```python
from build123d import *

# Parameters (mm, degrees)
SZKIC1_R                    = 1.5
SZKIC1_R_2                  = 1.6
DODANIE_WYCI_GNI_CIE1_DEPTH = 20
ZAOKR_GLENIE1_R             = 3
SFAZOWANIE1_SIZE            = 1
SZKIC2_R                    = 1.5
SZKIC2_R_2                  = 1.6
DODANIE_WYCI_GNI_CIE2_DEPTH = 0.2


with BuildPart() as part:
    # Szkic1 → Dodanie-wyciągnięcie1 (new body)
    with BuildSketch(Plane.XY):
        Polygon((-39.009773604, 35.733555733), (-39.009773604, 39.983555733), (9.235464557, 39.983555733), (9.235464557, 35.733555733), (9.235464557, -13.466444267), (9.235464557, -17.716444267), (-39.009773604, -17.716444267), (-39.009773604, -13.466444267), align=None)
        with Locations((5.112845476, 11.133555733)):
            Circle(SZKIC1_R, mode=Mode.SUBTRACT)
        with Locations((-34.887154524, 11.133555733)):
            Circle(SZKIC1_R, mode=Mode.SUBTRACT)
        with Locations((6.285464557, -13.466444267)):
            Circle(SZKIC1_R, mode=Mode.SUBTRACT)
        with Locations((6.285464557, 35.733555733)):
            Circle(SZKIC1_R_2, mode=Mode.SUBTRACT)
        with Locations((-36.059773604, 35.733555733)):
            Circle(SZKIC1_R, mode=Mode.SUBTRACT)
        with Locations((-36.059773604, -13.466444267)):
            Circle(SZKIC1_R, mode=Mode.SUBTRACT)
        with BuildLine():
            Line((-14.087154524, -13.391444267), (-14.087154524, -12.891444267))
            Line((-14.087154524, -12.891444267), (-3.372154524, -12.891444267))
            ThreePointArc((-3.372154524, -12.891444267), (-1.675098249, -12.188500541), (-0.972154524, -10.491444267))
            Line((-0.972154524, -10.491444267), (-0.972154524, -0.591444267))
            Line((-0.972154524, -0.591444267), (-0.472154524, -0.591444267))
            Line((-0.472154524, -0.591444267), (-0.472154524, 1.008555733))
            Line((-0.472154524, 1.008555733), (-0.972154524, 1.008555733))
            Line((-0.972154524, 1.008555733), (-0.972154524, 21.258555733))
            Line((-0.972154524, 21.258555733), (-0.472154524, 21.258555733))
            Line((-0.472154524, 21.258555733), (-0.472154524, 22.858555733))
            Line((-0.472154524, 22.858555733), (-0.972154524, 22.858555733))
            Line((-0.972154524, 22.858555733), (-0.972154524, 28.930128609))
            ThreePointArc((-0.972154524, 28.930128609), (-1.154843646, 29.848568846), (-1.675098249, 30.627184884))
            Line((-1.675098249, 30.627184884), (-5.503525374, 34.455612008))
            ThreePointArc((-5.503525374, 34.455612008), (-6.282141411, 34.975866612), (-7.200581648, 35.158555733))
            Line((-7.200581648, 35.158555733), (-14.087154524, 35.158555733))
            Line((-14.087154524, 35.158555733), (-14.087154524, 35.658555733))
            Line((-14.087154524, 35.658555733), (-15.687154524, 35.658555733))
            Line((-15.687154524, 35.658555733), (-15.687154524, 35.158555733))
            Line((-15.687154524, 35.158555733), (-22.573727399, 35.158555733))
            ThreePointArc((-22.573727399, 35.158555733), (-23.492167637, 34.975866612), (-24.270783674, 34.455612008))
            Line((-24.270783674, 34.455612008), (-28.099210798, 30.627184884))
            ThreePointArc((-28.099210798, 30.627184884), (-28.619465402, 29.848568846), (-28.802154524, 28.930128609))
            Line((-28.802154524, 28.930128609), (-28.802154524, 22.858555733))
            Line((-28.802154524, 22.858555733), (-29.302154524, 22.858555733))
            Line((-29.302154524, 22.858555733), (-29.302154524, 21.258555733))
            Line((-29.302154524, 21.258555733), (-28.802154524, 21.258555733))
            Line((-28.802154524, 21.258555733), (-28.802154524, 1.008555733))
            Line((-28.802154524, 1.008555733), (-29.302154524, 1.008555733))
            Line((-29.302154524, 1.008555733), (-29.302154524, -0.591444267))
            Line((-29.302154524, -0.591444267), (-28.802154524, -0.591444267))
            Line((-28.802154524, -0.591444267), (-28.802154524, -10.491444267))
            ThreePointArc((-28.802154524, -10.491444267), (-28.099210798, -12.188500541), (-26.402154524, -12.891444267))
            Line((-26.402154524, -12.891444267), (-15.687154524, -12.891444267))
            Line((-15.687154524, -12.891444267), (-15.687154524, -13.391444267))
            Line((-15.687154524, -13.391444267), (-14.087154524, -13.391444267))
        make_face(mode=Mode.SUBTRACT)
    extrude(amount=DODANIE_WYCI_GNI_CIE1_DEPTH)

    # Zaokrąglenie1
    zaokr_glenie1_edges = [part.edges().sort_by_distance(p)[0] for p in [
        (-39.009773604, 39.983555733, 10),
        (9.235464557, 39.983555733, 10),
        (9.235464557, -17.716444267, 10),
        (-39.009773604, -17.716444267, 10),
    ]]
    fillet(zaokr_glenie1_edges, radius=ZAOKR_GLENIE1_R)

    # Sfazowanie1
    sfazowanie1_edges = [part.edges().sort_by_distance(p)[0] for p in [
        (3.612845476, 11.133555733, 20),
        (-36.387154524, 11.133555733, 20),
    ]]
    chamfer(sfazowanie1_edges, length=SFAZOWANIE1_SIZE)

    # Szkic2 → Dodanie-wyciągnięcie2 (add)
    with BuildSketch(Plane(origin=(0, 0, 0), x_dir=(-1, 0, 0), z_dir=(0, 0, -1))):
        with Locations((36.059773604, 35.733555733)):
            Circle(SZKIC2_R)
        with Locations((34.887154524, 11.133555733)):
            Circle(SZKIC2_R)
        with Locations((36.059773604, -13.466444267)):
            Circle(SZKIC2_R)
        with Locations((-6.285464557, 35.733555733)):
            Circle(SZKIC2_R_2)
        with Locations((-5.112845476, 11.133555733)):
            Circle(SZKIC2_R)
        with Locations((-6.285464557, -13.466444267)):
            Circle(SZKIC2_R)
    extrude(amount=-DODANIE_WYCI_GNI_CIE2_DEPTH)


solid = part.part
```
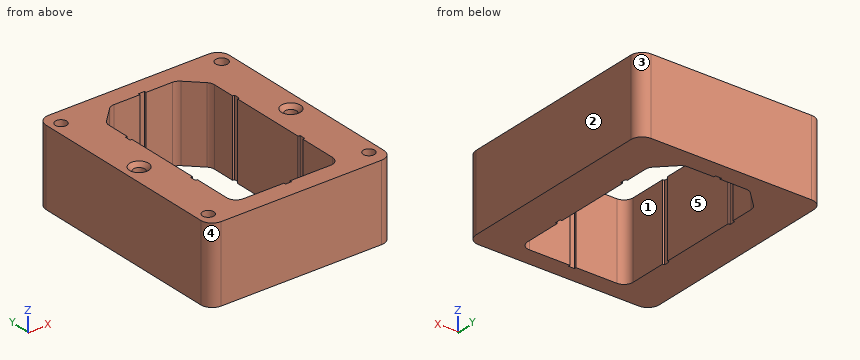
For this review, take the finished solid that the model builds, in its own axes (mm). Face numbers are marked on the shaded views. A direction names the side the tool comes from. Coordinates: 2 decimals unless noted, no trailing zeros. Loops run counter-clockwise (first coordinate to the right, second up) from the corner with the lowest first, then second, coordinate; pieces in that order, holes last.
1. Add section C-C, the plane z = 10.25. Count the separate pieces of the cut face and the enclosed holes in it, then the cut area to 3 significant figures.
2. For the marked faces 4 and 5, list the 3-axis set-ups (+Z, -Z, +X, -X, +Y, -Y) from which the entire face can be reached by the end or side of a thin tool; tool diameter is ignored.
3. Add section B-B, the plane y = 27. Give the boundary of the cut face in (x, z), then the cut area to 3 significant figures.
4. For line 1 (X direction, y = 19, z = 4.5); line 2 (Y direction, x = -15.5, z = 16); line 3 (Y direction, x = -19.5, z = 14.25), list the stretches that pass through material, from the lowest coordinate up.
5. Insertion check: P1, Ø1.5, axis at x = -36.5, y = -13, coming from the +Z side. The pin has a flat end and moves straight along its axis. Give the tip position at first contact, or say it passes through.
6. Mouldability with a two-part tool opening along Y and no side actions: class the marked faces 1, 2 and 3 as +Y half, -Y half, draft (parallel to the pull), parting line (faces both ways), or undercut.
7. Add section A-A, the plane x = -10.5. Give the boundary of the cut face in (y, z).
Result:
1. separate pieces: 1
1. enclosed holes: 7
1. area: 1,420 mm2
2. face 4: +Z, -Z, -X, -Y
2. face 5: +Z, -Z
3. outline: (-39.01, 0) - (-28.8, 0) - (-28.8, 20) - (-39.01, 20) - close; (-0.97, 0) - (9.24, 0) - (9.24, 20) - (-0.97, 20) - close
3. area: 408 mm2
4. line 1: x = -39.01 to -28.8, -0.97 to 9.24
4. line 2: y = -17.72 to -13.39, 35.66 to 39.98
4. line 3: y = -17.72 to -12.89, 35.16 to 39.98
5. P1: stops at z = 0.2
6. face 1: undercut
6. face 2: draft
6. face 3: +Y half
7. outline: (-17.72, 0) - (-12.89, 0) - (-12.89, 20) - (-17.72, 20) - close; (35.16, 0) - (39.98, 0) - (39.98, 20) - (35.16, 20) - close
